The model under review builds one solid part; all positions refer to its coordinate system, in mm. Round coordinates to 2 decimals unless told otherwise and drop trailing zeros. Order: outer loops, then holes, each group sorted by start corner. A loop starts at its lowest first (then second) coordinate and runs counter-clockwise, first axis right, second up. Notation, with made-up numbers: (-8.75, -38.75) - (-0.75, -38.75) arc R19 cw to (-0.75, -13.75) - close; hole circle Ø4 at (3, 47). An arc over 180 degrees is marked (long way). One line per question, with ' | ' between items. Start each with the question number.
Item 1: Add section B-B on x = 109. State the section outline as (y, z) points, and give its area (3 significant figures).
Item 2: Insertion check: pin 1 Ø2 at (x, z) = (123, 3) entering from -Y; pin 2 Ø1 at (y, z) = (12, 1.5) entering from -X; pin 3 Ø1 at (x, z) = (93.5, 1) entering from -Y; pin 4 Ø1.5 at (x, y) = (32, -53.5) entering from -Z. Each pin has a flat end and moves straight along its axis. Give the tip position at first contact, or say it passes through.
Item 3: Add section A-A on y = -28. State the section outline as (x, z) points, and give its area (3 significant figures).
Item 4: For L1, parallel to Y at x = 56.5, z = 1.6; L2, parallel to Y at x = 77, z = 2.65; L3, parallel to Y at x = 108, z = 3.5, list the stretches that pass through material, from the lowest coordinate up. Write a range as [from, to].
Item 5: Add section C-C on y = -42.5. State the section outline as (x, z) points.
from build123d import *

# Parameters (mm, degrees)
BOSS_EXTRUDE1_DEPTH = 4
FILLET1_R           = 10
FILLET2_R           = 5
CUT_EXTRUDE1_DEPTH  = 4
LPATTERN1_COUNT     = 3
LPATTERN1_PITCH     = 8
FILLET3_R           = 2
FILLET4_R           = 2
CUT_EXTRUDE2_DEPTH  = 10
FILLET5_R           = 2
FILLET6_R           = 1


with BuildPart() as part:
    # Sketch1 → Boss-Extrude1 (new body)
    with BuildSketch(Plane.XY):
        Polygon((10, 0), (-2.34288865, -70), (37.65711135, -70), (43.652228694, -36), (85.284719782, -36), (91.632491087, 0), (145, 0), (145, 20), (140, 20), (140, 25), (145, 25), (145, 30), (0, 30), (0, 0), align=None)
        Polygon((44.710190579, -30), (80.250121995, -30), (85.539931416, 0), (50, 0), align=None, mode=Mode.SUBTRACT)
    extrude(amount=BOSS_EXTRUDE1_DEPTH)

    # Fillet1
    # the kernel refuses this fillet: 10 mm, written as the material it adds along each edge
    with BuildSketch(Plane(origin=(10, 0, 0), x_dir=(-0.17364817766693433, -0.9848077530122074, 0), z_dir=(0, 0, 1))) as fillet1_piece_1:
        with BuildLine():
            CenterArc((11.735327688, -10), FILLET1_R, 90, 89.129514879)
            Line((1.736481777, -9.84807753), (1.536504858, -9.845039081))
            ThreePointArc((1.536504858, -9.845039081), (0.671279338, -4.958768401), (-0.196961551, -0.034729636))
            Line((-0.196961551, -0.034729636), (0, 0.2))
            Line((0, 0.2), (11.735327688, 0.2))
            Line((11.735327688, 0.2), (11.735327688, 0))
        make_face()
    extrude(amount=4)

    # Fillet2
    fillet2_edges = [part.edges().sort_by_distance(p)[0] for p in [
        (145, 0, 2),
        (91.632491087, 0, 2),
        (85.284719782, -36, 2),
        (43.652228694, -36, 2),
        (37.65711135, -70, 2),
        (-2.34288865, -70, 2),
        (85.539931416, 0, 2),
        (50, 0, 2),
        (44.710190579, -30, 2),
        (80.250121995, -30, 2),
    ]]
    fillet(fillet2_edges, radius=FILLET2_R)

    # Sketch2 → Cut-Extrude1 (cut)
    with BuildSketch(Plane.XY.offset(4)):
        Polygon((0, 20), (0, 28), (5, 27), align=None)
    cut_extrude1 = extrude(amount=-CUT_EXTRUDE1_DEPTH, mode=Mode.SUBTRACT)

    # LPattern1: Cut-Extrude1 ×3
    with Locations(*[(0, -i * LPATTERN1_PITCH, 0) for i in range(1, LPATTERN1_COUNT)]):
        add(cut_extrude1, mode=Mode.SUBTRACT)

    # Fillet3
    fillet3_edges = [part.edges().sort_by_distance(p)[0] for p in [
        (145, 25, 2),
        (140, 25, 2),
        (140, 20, 2),
        (145, 20, 2),
    ]]
    fillet(fillet3_edges, radius=FILLET3_R)

    # Fillet4
    fillet4_edges = [part.edges().sort_by_distance(p)[0] for p in [
        (145, 30, 2),
    ]]
    fillet(fillet4_edges, radius=FILLET4_R)

    # Sketch3 → Cut-Extrude2 (cut)
    with BuildSketch(Plane.XY.offset(4)):
        Polygon((3.410578707, 27.317884259), (3.410578707, 32.702988903), (-2.245047392, 32.702988903), (-2.245047392, 26.199863932), align=None)
    extrude(amount=-CUT_EXTRUDE2_DEPTH, mode=Mode.SUBTRACT)

    # Fillet5
    fillet5_edges = [part.edges().sort_by_distance(p)[0] for p in [
        (3.410578707, 30, 2),
    ]]
    fillet(fillet5_edges, radius=FILLET5_R)

    # Fillet6
    fillet6_edges = [part.edges().sort_by_distance(p)[0] for p in [
        (3.410578707, 27.317884259, 2),
    ]]
    fillet(fillet6_edges, radius=FILLET6_R)


solid = part.part
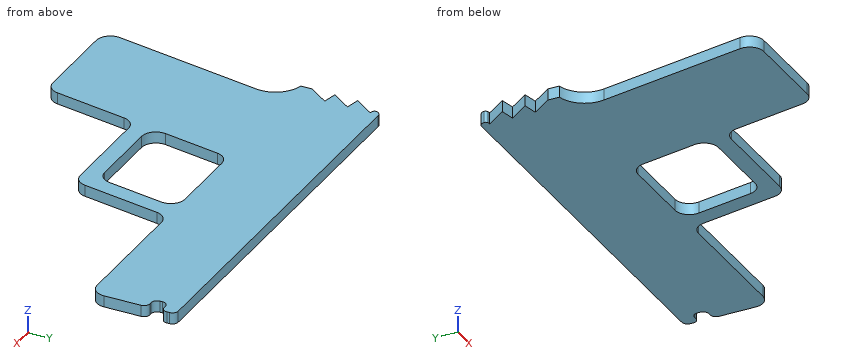
Determined:
1) outline: (0, 0) - (30, 0) - (30, 4) - (0, 4) - close | area: 120 mm2
2) pin 1: y = 0 | pin 2: x = 0 | pin 3: y = -0.88 | pin 4: z = 0
3) outline: (5.06, 0) - (46.67, 0) - (46.67, 4) - (5.06, 4) - close; (80.05, 0) - (86.7, 0) - (86.7, 4) - (80.05, 4) - close | area: 193 mm2
4) L1: [-36, -30], [0, 30] | L2: [-36, -29.91], [0, 30] | L3: [0, 30]
5) outline: (2.51, 0) - (42.51, 0) - (42.51, 4) - (2.51, 4) - close
